from build123d import *

# Parameters (mm, degrees)
SKETCH1_W           = 24
SKETCH1_H           = 60
BOSS_EXTRUDE1_DEPTH = 36.8
CUT_EXTRUDE1_DEPTH  = 54.2
CUT_EXTRUDE2_DEPTH  = 54.2
SKETCH4_R           = 1.2
CUT_EXTRUDE3_DEPTH  = 53.690630097
SKETCH5_W           = 54
SKETCH5_H           = 25.8
CUT_EXTRUDE4_DEPTH  = 54.2
SKETCH6_W           = 24
SKETCH6_H           = 3
BOSS_EXTRUDE2_DEPTH = 9
SKETCH7_W           = 24
SKETCH7_H           = 3
BOSS_EXTRUDE3_DEPTH = 9
SKETCH8_R           = 1.7
CUT_EXTRUDE5_DEPTH  = 6
SKETCH9_W           = 4
SKETCH9_H           = 20
CUT_EXTRUDE6_DEPTH  = 17
CHAMFER1_SIZE       = 6.5


with BuildPart() as part:
    # Sketch1 → Boss-Extrude1 (new body)
    with BuildSketch(Plane(origin=(0, 0, 0), x_dir=(1, 0, 0), z_dir=(0, 1, 0))):
        Rectangle(SKETCH1_W, SKETCH1_H)
    extrude(amount=BOSS_EXTRUDE1_DEPTH)

    # Sketch2 → Cut-Extrude1 (cut, through all)
    with BuildSketch(Plane(origin=(12, 0, 0), x_dir=(0, 0, -1), z_dir=(1, 0, 0))):
        with BuildLine():
            Line((-12.75, 36.8), (-12.75, 32.424807681))
            ThreePointArc((-12.75, 32.424807681), (-12.25, 29.1), (-11.75, 32.424807681))
            Line((-11.75, 32.424807681), (-11.75, 36.8))
            Line((-11.75, 36.8), (-12.75, 36.8))
        make_face()
        with BuildLine():
            Line((-8.25, 32.424807681), (-8.25, 36.8))
            Line((-8.25, 36.8), (-7.25, 36.8))
            Line((-7.25, 36.8), (-7.25, 32.424807681))
            ThreePointArc((-7.25, 32.424807681), (-7.75, 29.1), (-8.25, 32.424807681))
        make_face()
    extrude(amount=-CUT_EXTRUDE1_DEPTH, mode=Mode.SUBTRACT)

    # Sketch3 → Cut-Extrude2 (cut, through all)
    with BuildSketch(Plane(origin=(12, 0, 0), x_dir=(0, 0, -1), z_dir=(1, 0, 0))):
        with BuildLine():
            Line((-14.25, 36.8), (-14.25, 33.297999199))
            ThreePointArc((-14.25, 33.297999199), (-15.430565736, 31.152138611), (-14.747999199, 28.8))
            Line((-14.747999199, 28.8), (-30, 28.8))
            Line((-30, 28.8), (-30, 36.8))
            Line((-30, 36.8), (-14.25, 36.8))
        make_face()
        with BuildLine():
            Line((30, 28.8), (30, 36.8))
            Line((30, 36.8), (-5.75, 36.8))
            Line((-5.75, 36.8), (-5.75, 33.297999199))
            ThreePointArc((-5.75, 33.297999199), (-4.569434264, 31.152138611), (-5.252000801, 28.8))
            Line((-5.252000801, 28.8), (30, 28.8))
        make_face()
    extrude(amount=-CUT_EXTRUDE2_DEPTH, mode=Mode.SUBTRACT)

    # Sketch4 → Cut-Extrude3 (cut, through all)
    with BuildSketch(Plane(origin=(0, 0, 5.75), x_dir=(-1, 0, 0), z_dir=(0, 0, -1))):
        with Locations((-5, 35.0489996)):
            Circle(SKETCH4_R)
        with Locations((5, 35.0489996)):
            Circle(SKETCH4_R)
    extrude(amount=-CUT_EXTRUDE3_DEPTH, mode=Mode.SUBTRACT)

    # Sketch5 → Cut-Extrude4 (cut, through all)
    with BuildSketch(Plane(origin=(12, 0, 0), x_dir=(0, 0, -1), z_dir=(1, 0, 0))):
        with Locations((0, 12.9)):
            Rectangle(SKETCH5_W, SKETCH5_H)
    extrude(amount=-CUT_EXTRUDE4_DEPTH, mode=Mode.SUBTRACT)

    # Sketch6 → Boss-Extrude2 (add)
    with BuildSketch(Plane(origin=(0, 0, -30), x_dir=(-1, 0, 0), z_dir=(0, 0, -1))):
        with Locations((0, 1.5)):
            Rectangle(SKETCH6_W, SKETCH6_H)
    extrude(amount=-BOSS_EXTRUDE2_DEPTH)

    # Sketch7 → Boss-Extrude3 (add)
    with BuildSketch(Plane.XY.offset(30)):
        with Locations((0, 1.5)):
            Rectangle(SKETCH7_W, SKETCH7_H)
    extrude(amount=-BOSS_EXTRUDE3_DEPTH)

    # Sketch8 → Cut-Extrude5 (cut)
    with BuildSketch(Plane(origin=(0, 3, 0), x_dir=(1, 0, 0), z_dir=(0, 1, 0))):
        with Locations(Location((-5, 23.6, 0), (0, 0, 180))):
            Circle(SKETCH8_R)
        with Locations(Location((5, 23.6, 0), (0, 0, 180))):
            Circle(SKETCH8_R)
        with Locations(Location((-5, -23.6, 0), (0, 0, 180))):
            Circle(SKETCH8_R)
        with Locations(Location((5, -23.6, 0), (0, 0, 180))):
            Circle(SKETCH8_R)
    extrude(amount=-CUT_EXTRUDE5_DEPTH, mode=Mode.SUBTRACT)

    # Sketch9 → Cut-Extrude6 (cut)
    with BuildSketch(Plane.XY.offset(30)):
        with Locations((0, 10)):
            Rectangle(SKETCH9_W, SKETCH9_H)
    extrude(amount=-CUT_EXTRUDE6_DEPTH, mode=Mode.SUBTRACT)

    # Chamfer1
    # the kernel refuses this chamfer: 6.5 mm, written as the material it adds along each edge
    with BuildSketch(Plane(origin=(12, 25.8, -27), x_dir=(0, -0.9996219169112968, -0.027495876610587486), z_dir=(-1, 0, 0))) as chamfer1_piece_1:
        Polygon((CHAMFER1_SIZE * 0.999621916911, CHAMFER1_SIZE * 0.0274958766106), (-CHAMFER1_SIZE * 0.0274958766106, CHAMFER1_SIZE * 0.999621916911), (0, 0), align=None)
    extrude(amount=24)
    with BuildSketch(Plane(origin=(12, 25.8, 27), x_dir=(0, -0.9996219169112968, 0.027495876610586424), z_dir=(-1, 0, 0))) as chamfer1_piece_2_section:
        Polygon((CHAMFER1_SIZE * 0.999621916911, -CHAMFER1_SIZE * 0.0274958766106), (-CHAMFER1_SIZE * 0.0274958766106, -CHAMFER1_SIZE * 0.999621916911), (0, 0), align=None)
    chamfer1_piece_2 = extrude(amount=24, mode=Mode.PRIVATE)
    chamfer1_piece_2 = split(chamfer1_piece_2, bisect_by=Plane(origin=(7, 20, 26.950497718), z_dir=(0, -1, 0)), keep=Keep.TOP, mode=Mode.PRIVATE)
    chamfer1_piece_2 = split(chamfer1_piece_2, bisect_by=Plane(origin=(2, 19.670055839, 26.950497718), z_dir=(1, 0, 0)), keep=Keep.TOP, mode=Mode.PRIVATE)
    add(chamfer1_piece_2)
    with BuildSketch(Plane(origin=(12, 25.8, 27), x_dir=(0, -0.9996219169112968, 0.027495876610586424), z_dir=(-1, 0, 0))) as chamfer1_piece_3_section:
        Polygon((CHAMFER1_SIZE * 0.999621916911, -CHAMFER1_SIZE * 0.0274958766106), (-CHAMFER1_SIZE * 0.0274958766106, -CHAMFER1_SIZE * 0.999621916911), (0, 0), align=None)
    chamfer1_piece_3 = extrude(amount=24, mode=Mode.PRIVATE)
    chamfer1_piece_3 = split(chamfer1_piece_3, bisect_by=Plane(origin=(7, 20, 24.812647942), z_dir=(0, 1, 0)), keep=Keep.TOP, mode=Mode.PRIVATE)
    chamfer1_piece_3 = split(chamfer1_piece_3, bisect_by=Plane(origin=(2, 23.739513204, 24.812647942), z_dir=(1, 0, 0)), keep=Keep.TOP, mode=Mode.PRIVATE)
    add(chamfer1_piece_3)
    with BuildSketch(Plane(origin=(12, 25.8, 27), x_dir=(0, -0.9996219169112968, 0.027495876610586424), z_dir=(-1, 0, 0))) as chamfer1_piece_4_section:
        Polygon((CHAMFER1_SIZE * 0.999621916911, -CHAMFER1_SIZE * 0.0274958766106), (-CHAMFER1_SIZE * 0.0274958766106, -CHAMFER1_SIZE * 0.999621916911), (0, 0), align=None)
    chamfer1_piece_4 = extrude(amount=24, mode=Mode.PRIVATE)
    chamfer1_piece_4 = split(chamfer1_piece_4, bisect_by=Plane(origin=(-2, 23.739513204, 24.812647942), z_dir=(1, 0, 0)), keep=Keep.TOP, mode=Mode.PRIVATE)
    chamfer1_piece_4 = split(chamfer1_piece_4, bisect_by=Plane(origin=(0, 20, 24.812647942), z_dir=(0, 1, 0)), keep=Keep.TOP, mode=Mode.PRIVATE)
    chamfer1_piece_4 = split(chamfer1_piece_4, bisect_by=Plane(origin=(2, 23.739513204, 24.812647942), z_dir=(-1, 0, 0)), keep=Keep.TOP, mode=Mode.PRIVATE)
    add(chamfer1_piece_4)
    with BuildSketch(Plane(origin=(12, 25.8, 27), x_dir=(0, -0.9996219169112968, 0.027495876610586424), z_dir=(-1, 0, 0))) as chamfer1_piece_5_section:
        Polygon((CHAMFER1_SIZE * 0.999621916911, -CHAMFER1_SIZE * 0.0274958766106), (-CHAMFER1_SIZE * 0.0274958766106, -CHAMFER1_SIZE * 0.999621916911), (0, 0), align=None)
    chamfer1_piece_5 = extrude(amount=24, mode=Mode.PRIVATE)
    chamfer1_piece_5 = split(chamfer1_piece_5, bisect_by=Plane(origin=(-2, 19.670055839, 26.950497718), z_dir=(-1, 0, 0)), keep=Keep.TOP, mode=Mode.PRIVATE)
    chamfer1_piece_5 = split(chamfer1_piece_5, bisect_by=Plane(origin=(-7, 20, 26.950497718), z_dir=(0, -1, 0)), keep=Keep.TOP, mode=Mode.PRIVATE)
    add(chamfer1_piece_5)
    with BuildSketch(Plane(origin=(12, 25.8, 27), x_dir=(0, -0.9996219169112968, 0.027495876610586424), z_dir=(-1, 0, 0))) as chamfer1_piece_6_section:
        Polygon((CHAMFER1_SIZE * 0.999621916911, -CHAMFER1_SIZE * 0.0274958766106), (-CHAMFER1_SIZE * 0.0274958766106, -CHAMFER1_SIZE * 0.999621916911), (0, 0), align=None)
    chamfer1_piece_6 = extrude(amount=24, mode=Mode.PRIVATE)
    chamfer1_piece_6 = split(chamfer1_piece_6, bisect_by=Plane(origin=(-2, 23.739513204, 24.812647942), z_dir=(-1, 0, 0)), keep=Keep.TOP, mode=Mode.PRIVATE)
    chamfer1_piece_6 = split(chamfer1_piece_6, bisect_by=Plane(origin=(-7, 20, 24.812647942), z_dir=(0, 1, 0)), keep=Keep.TOP, mode=Mode.PRIVATE)
    add(chamfer1_piece_6)


solid = part.part
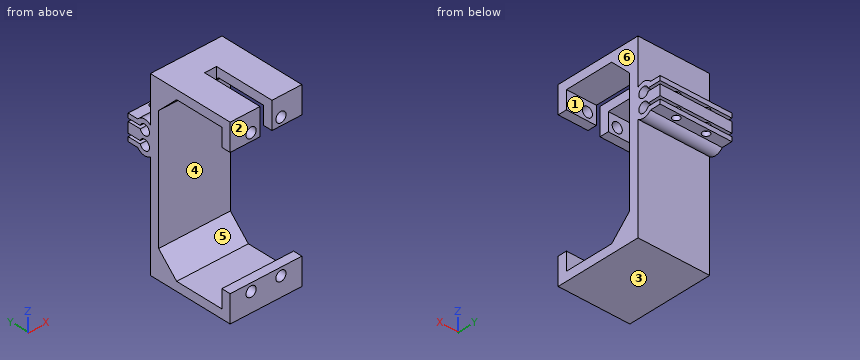
Geometry: final body of the model. Coordinates: model frame, mm. Face numbers are marked on the shaded views. A direction names the side the tool comes from. Coordinates: 2 decimals unless noted, no trailing zeros. Order: outer loops, then holes, each group sorted by start corner. A loop starts at its lowest first (then second) coordinate and runs counter-clockwise, first axis right, second up. Notation, with made-up numbers: (-0.5, 70) - (50.5, 70) arc R34 cw to (50.5, 109) - close; hole circle Ø5 at (19.5, -29.5). An arc over 180 degrees is marked (long way). Use one line per item in the form item = value.
1) Section D-D (x = 0.75). Return loops of the section in (y, z), then the cut area to 3 significant figures.
Solutions:
outline = (0, -30) - (28.8, -30) - (28.8, 5.25) arc R3.2 ccw to (33.3, 5.75) - (36.8, 5.75) - (36.8, 7.25) - (32.42, 7.25) arc R1.7 cw (long way) to (32.42, 8.25) - (36.8, 8.25) - (36.8, 11.75) - (32.42, 11.75) arc R1.7 cw (long way) to (32.42, 12.75) - (36.8, 12.75) - (36.8, 14.25) - (33.3, 14.25) arc R3.2 ccw to (28.8, 14.75) - (28.8, 30) - (20, 30) - (20, 26.3) - (25.8, 20.5) - (25.8, -20.5) - (19.3, -27) - (3, -27) - (3, -21) - (0, -21) - close
area = 384 mm^2
2) Pin query (flat end, axial travel): pin 1 (3.5 mm diameter, centred on x = -1, y = 35.5, fed in from +Z); pin 2 (4 mm diameter, centred on y = 31, z = 2.5, fed in from -X) (3 decimals); pin 3 (3 mm diameter, centred on x = 5, y = 35.049, fed in from -Z); pin 4 (4 mm diameter, centred on x = -5, y = 35.049, fed in from +Z). Return the tip coordinate at first contact, or that it passes through.
Solutions:
pin_1 = 14.25
pin_2 = through
pin_3 = 5.75
pin_4 = 14.53
3) Section A-A (y = 14). Return loops of the section in (x, z), then the cut area to 3 significant figures.
Solutions:
outline = (-12, -30) - (12, -30) - (12, -27) - (-12, -27) - close; (-12, 27) - (-2, 27) - (-2, 30) - (-12, 30) - close; (2, 27) - (12, 27) - (12, 30) - (2, 30) - close
area = 132 mm^2
4) Section B-B (z = -23.6). Return loops of the section in (x, y), then the cut area to 3 significant figures.
Solutions:
outline = (-12, 0) - (-6.7, 0) - (-6.7, 3) - (-12, 3) - close; (-12, 22.7) - (12, 22.7) - (12, 28.8) - (-12, 28.8) - close; (-3.3, 0) - (3.3, 0) - (3.3, 3) - (-3.3, 3) - close; (6.7, 0) - (12, 0) - (12, 3) - (6.7, 3) - close
area = 198 mm^2
5) Set-up query: the marked faces 4, 5 and 6. Return all of +Z, -Z, +X, -X, +Y, -Y with unobstructed straight access to the full face (end or side cutting, diameter ignored); none if empty.
Solutions:
face_4 = +X, -X, -Y
face_5 = +X, -X
face_6 = +Z, -Z, +X, +Y, -Y
6) Mould query, pull axis Y, two halves, no side actions, for the marked faces 1, 2 and 3. Classes: +Y half, -Y half, draft (parallel to the pull), parting line (faces both ways), or undercut.
Solutions:
face_1 = undercut
face_2 = -Y half
face_3 = draft
7) Ray query, L1, parallel to Z at x = 0.5, y = 35; L2, parallel to Z at x = -5, y = 2; L3, parallel to Z at x = 5.25, y = 30.8. Return the intervals inside material, ascending.
Solutions:
L1 = 5.75 to 7.25, 8.25 to 11.75, 12.75 to 14.25
L2 = -30 to -25.3, -21.9 to -21, 21 to 21.9, 25.3 to 30
L3 = 4.55 to 6.05, 9.45 to 10.55, 13.95 to 15.45
8) Section C-C (y = 25). Return loops of the section in (x, z).
Solutions:
outline = (-12, -30) - (12, -30) - (12, -21.3) - (-12, -21.3) - close; (-12, 21.3) - (12, 21.3) - (12, 30) - (-12, 30) - close
